Work out the finished part from the listing and answer in its coordinate system (mm). Give positions to 0.01 mm unless a question says otherwise; leave off trailing zeros. Write each loop counter-clockwise with the first axis right and the second up, starting at its lowest first coordinate (ties: lowest second). Pieces come first, ordered by that corner, then holes.
1) Find section B-B (x = 24.5). Determine the outline of the cut face in (y, z).
2) A straight line is drawn through the part: probe 1 along Y at (x, z) = (9.5, 28). Find the intervals that lie inside material, in ascending order.
3) Find section C-C (z = 7). Determine the outline of the cut face in (x, y).
4) Given pin 1 Ø0.8 at (x, y) = (-54, 4) entering from -Z; pin 2 Ø2 at (y, z) = (4.5, -45.5) entering from +X; pin 3 Ø6 at (x, z) = (-43.5, -0.5) entering from +Y, each flat-ended and moving along its own axis, determine where each tip first touches the part or whether it passes through.
5) Find section A-A (y = 3.85). Determine the outline of the cut face in (x, z).
```python
from build123d import *

# Parameters (mm, degrees)
SKETCH1_W           = 118
SKETCH1_H           = 100
BOSS_EXTRUDE1_DEPTH = 3
FILLET1_R           = 2
SKETCH2_W           = 3.5
SKETCH2_H           = 2.5
BOSS_EXTRUDE2_DEPTH = 2.5


with BuildPart() as part:
    # Sketch1 → Boss-Extrude1 (new body)
    with BuildSketch(Plane(origin=(0, 0, 0), x_dir=(1, 0, 0), z_dir=(0, 1, 0))):
        Rectangle(SKETCH1_W, SKETCH1_H)
    extrude(amount=BOSS_EXTRUDE1_DEPTH)

    # Fillet1
    fillet1_edges = [part.edges().sort_by_distance(p)[0] for p in [
        (59, 1.5, 50),
        (-59, 1.5, 50),
        (-59, 1.5, -50),
        (59, 1.5, -50),
    ]]
    fillet(fillet1_edges, radius=FILLET1_R)

    # Sketch2 → Boss-Extrude2 (add)
    with BuildSketch(Plane(origin=(0, 3, 0), x_dir=(1, 0, 0), z_dir=(0, 1, 0))):
        with Locations((-54, -34)):
            Rectangle(SKETCH2_W, SKETCH2_H)
        with Locations((54, -34)):
            Rectangle(SKETCH2_W, SKETCH2_H)
        with Locations((0, 45)):
            Rectangle(SKETCH2_W, SKETCH2_H)
    extrude(amount=BOSS_EXTRUDE2_DEPTH)


solid = part.part
```
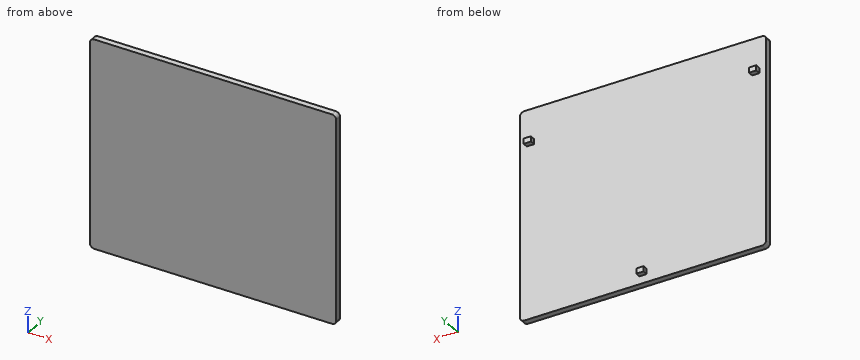
Results:
1. outline: (0, -50) - (3, -50) - (3, 50) - (0, 50) - close
2. probe 1: y = 0 to 3
3. outline: (-59, 0) - (59, 0) - (59, 3) - (-59, 3) - close
4. pin 1: stops at z = 32.75
4. pin 2: stops at x = 1.75
4. pin 3: stops at y = 3
5. outline: (-55.75, 32.75) - (-52.25, 32.75) - (-52.25, 35.25) - (-55.75, 35.25) - close; (-1.75, -46.25) - (1.75, -46.25) - (1.75, -43.75) - (-1.75, -43.75) - close; (52.25, 32.75) - (55.75, 32.75) - (55.75, 35.25) - (52.25, 35.25) - close
